Part model, mm, in its own coordinate system. Face numbers are marked on the shaded views. A direction names the side the tool comes from. Give positions to 0.01 mm unless a question says otherwise; leave off trailing zeros. Write each loop counter-clockwise with the first axis right and the second up, starting at its lowest first coordinate (ties: lowest second). Pieces come first, ordered by that corner, then holes. Notation, with made-up numbers: (70, 18.25) - (103, 18.25) arc R20 cw to (103, 45.25) - close; hole circle Ø2 at (88.5, -24.75). An arc over 180 degrees is marked (long way). Answer as a JSON object with one key per item and string values. Group by question number.
```python
from build123d import *

# Parameters (mm, degrees)
BOSS_EXTRUDE1_DEPTH         = 2.54
BOSS_EXTRUDE2_DEPTH         = 25.4
F_1_4_0_25_DIAMETER_HOLE1_D = 6.35


with BuildPart() as part:
    # Sketch1 → Boss-Extrude1 (new body)
    with BuildSketch(Plane(origin=(0, 0, 0), x_dir=(1, 0, 0), z_dir=(0, 1, 0))):
        Polygon((-26.320348586, -42.4), (-50.8, 0), (-25.4, 0), (-15.585045424, -17), (15.585045424, -17), (25.4, 0), (50.8, 0), (26.320348586, -42.4), align=None)
    extrude(amount=BOSS_EXTRUDE1_DEPTH)

    # Sketch2 → Boss-Extrude2 (add)
    with BuildSketch(Plane(origin=(0, 2.54, 0), x_dir=(1, 0, 0), z_dir=(0, 1, 0))):
        Polygon((-26.320348586, -42.4), (-15.585045424, -17), (-13.045045424, -17), (-13.045045424, -42.4), align=None)
        Polygon((15.585045424, -17), (26.320348586, -42.4), (13.045045424, -42.4), (13.045045424, -17), align=None)
    extrude(amount=BOSS_EXTRUDE2_DEPTH)

    # 1/4 (0.25) Diameter Hole1 (through all)
    with Locations(Plane(origin=(29.526348503, 2.54, 14.85), x_dir=(0, 0, 1), z_dir=(0, 1, 0))):
        with Locations((0, 0), (0, -59.052697006)):
            Hole(F_1_4_0_25_DIAMETER_HOLE1_D / 2)


solid = part.part
```
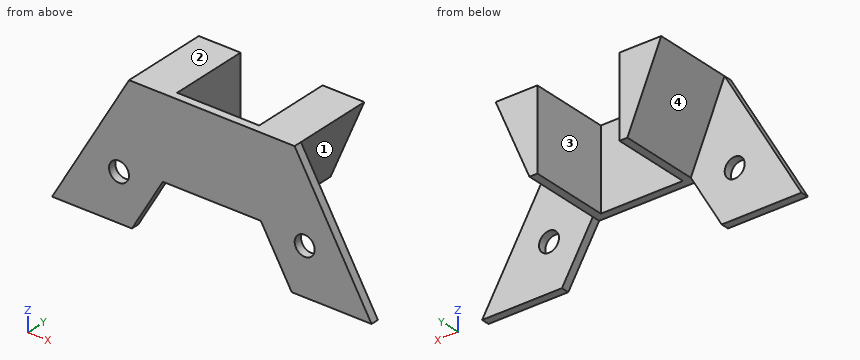
1) Saw through at D-D (z = 23). List the corners of the cut face in (x, y).
2) Saw through at B-B (z = 7). List the corners of the cut face in (x, y), and give its area (3 significant figures).
3) Saw through at C-C (z = 14.85). List the corners of the cut face in (x, y), and give its area (3 significant figures).
4) Which spindle directions (+Z, -Z, +X, -X, +Y, -Y) get a long thin tool onto all of the face, cutting with end or side? Do the marked faces 1, 2, 3 and 4. Say none if no direction does.
5) Drop flat-ended pins along their axis: P1, Ø12.5, axis at x = 0.5, z = 25, coming from the +Y side; P2, Ø14, axis at x = -6.5, y = 12.5, coming from the -Z side; P3, Ø4, axis at y = 19.5, z = 22.5, coming from the +X side; P4, Ø1, axis at x = -32.5, z = 11, coming from the -Y side. Give the stop position or say it passes through.
6) Drill centre lines: line 1 along X through (y, z) = (0.65, 14.85); line 2 along Y through (x, z) = (7, 28); line 3 along X through (y, z) = (22.5, 21). Where is each one in solid material? Low to high. Write a range as from..to.
7) Saw through at A-A (y = 21.5). List the corners of the cut face in (x, z).
Checks:
{
 "1": {"outline": "(-37.52, 0) - (37.52, 0) - (37.52, 2.54) - (18.12, 2.54) - (18.12, 27.94) - (13.05, 27.94) - (13.05, 2.54) - (-13.05, 2.54) - (-13.05, 27.94) - (-18.12, 27.94) - (-18.12, 2.54) - (-37.52, 2.54) - close"},
 "2": {"outline": "(-46.76, 0) - (-21.36, 0) - (-21.36, 2.54) - (-46.76, 2.54) - close; (21.36, 0) - (46.76, 0) - (46.76, 2.54) - (21.36, 2.54) - close", "area": "129 mm2"},
 "3": {"outline": "(-42.23, 0) - (-32.7, 0) - (-32.7, 2.54) - (-42.23, 2.54) - close; (-26.35, 0) - (-16.83, 0) - (-16.83, 2.54) - (-26.35, 2.54) - close; (16.83, 0) - (26.35, 0) - (26.35, 2.54) - (16.83, 2.54) - close; (32.7, 0) - (42.23, 0) - (42.23, 2.54) - (32.7, 2.54) - close", "area": "96.8 mm2"},
 "4": {"face 1": "-Z, +X, +Y", "face 2": "+Z, +X, -X, +Y, -Y", "face 3": "+Z, -Z, +Y", "face 4": "-Z, -X, +Y"},
 "5": {"P1": "y = 2.54", "P2": "z = 17", "P3": "x = 18.75", "P4": "y = 0"},
 "6": {"line 1": "-42.23..-32.7, -26.35..-16.83, 16.83..26.35, 32.7..42.23", "line 2": "0..2.54", "line 3": "-17.28..-13.05, 13.05..17.28"},
 "7": {"outline": "(-26.32, 42.4) - (-15.59, 17) - (-13.05, 17) - (-13.05, 42.4) - close; (13.05, 17) - (15.59, 17) - (26.32, 42.4) - (13.05, 42.4) - close"}
}
